from build123d import *

# Parameters (mm, degrees)
BOSS_EXTRUDE1_DEPTH           = 17
CUT_EXTRUDE1_DEPTH            = 17
SKETCH3_R                     = 1.25
CUT_EXTRUDE2_DEPTH            = 17
CUT_EXTRUDE3_START            = -10.402815
SKETCH4_W                     = 3.3
SKETCH4_H                     = 12.499682623
CUT_EXTRUDE3_DEPTH            = 10.402815
SKETCH5_R                     = 2.25
SKETCH5_R_2                   = 1.25
EXTRUDE_THIN1_DEPTH           = 1.65
EXTRUDE_THIN1_TAPER           = -30
EXTRUDE_THIN1_OTHER_WAY_DEPTH = 1.65
EXTRUDE_THIN1_OTHER_WAY_TAPER = -30
SKETCH6_R                     = 1.25
CUT_EXTRUDE4_DEPTH            = 58.713758796
CUT_EXTRUDE5_DEPTH            = 47
CUT_EXTRUDE6_DEPTH            = 51
SKETCH9_R                     = 4
CUT_EXTRUDE7_DEPTH            = 51
CHAMFER2_SIZE                 = 4
CHAMFER2_SIZE_2               = 0.5
FILLET3_R                     = 30
FILLET4_SIZE                  = 2
FILLET4_SIZE_2                = 10


with BuildPart() as part:
    # Sketch1 → Boss-Extrude1 (new body)
    with BuildSketch(Plane.XY):
        Polygon((0, 0), (-3.159113316, 10.05), (-6.746853749, 9.105426772), (-9.395430715, 19.165426772), (-16.396843313, 17.322108667), (-13.748266347, 7.262108667), (-16.987870242, 6.409192141), (-13.249821349, -13.430807859), (-10.069194805, -33.377281726), (4.664340434, -45.432247006), (8.210516928, -41.098122841), (1.353313338, -35.487565032), (13.657279278, -20.449702081), (20.514482868, -26.06025989), (24.060659362, -21.726135725), (15.88, -15.032727593), align=None)
    extrude(amount=BOSS_EXTRUDE1_DEPTH)

    # Sketch2 → Cut-Extrude1 (cut)
    with BuildSketch(Plane(origin=(-11.069057434, -2.914239618, 0), x_dir=(0, 0, 1), z_dir=(-0.9670459389139427, -0.2546019482055291, 0))):
        with BuildLine():
            Line((14.33099337, 13.694095472), (13.19, 10.523128091))
            Line((13.19, 10.523128091), (20.415721384, 10.523128091))
            Line((20.415721384, 10.523128091), (20.415721384, 21.928823046))
            Line((20.415721384, 21.928823046), (-2.093019815, 21.928823046))
            Line((-2.093019815, 21.928823046), (-2.093019815, 20.981086575))
            Line((-2.093019815, 20.981086575), (9.161350785, 20.925943092))
            ThreePointArc((9.161350785, 20.925943092), (13.295140538, 18.417290029), (14.33099337, 13.694095472))
        make_face()
    extrude(amount=-CUT_EXTRUDE1_DEPTH, mode=Mode.SUBTRACT)

    # Sketch3 → Cut-Extrude2 (cut)
    with BuildSketch(Plane(origin=(-11.069057434, -2.914239618, 0), x_dir=(0, 0, 1), z_dir=(-0.9670459389139427, -0.2546019482055291, 0))):
        with Locations(Location((8.8, 16.925943092, 0), (0, 0, 270))):
            Circle(SKETCH3_R)
    extrude(amount=-CUT_EXTRUDE2_DEPTH, mode=Mode.SUBTRACT)

    # Sketch4 → Cut-Extrude3 (cut)
    with BuildSketch(Plane(origin=(-5.327785879, 20.236348285, 0), x_dir=(0.9670459389139427, 0.2546019482055291, 0), z_dir=(-0.2546019482055291, 0.9670459389139427, 0)).offset(CUT_EXTRUDE3_START)):
        with Locations((-7.826258123, -8.749841312)):
            Rectangle(SKETCH4_W, SKETCH4_H)
    extrude(amount=CUT_EXTRUDE3_DEPTH, mode=Mode.SUBTRACT)

    # Sketch5 → Extrude-Thin1 (add)
    with BuildSketch(Plane(origin=(-7.568351135, -1.992580565, 0), x_dir=(0, 0, 1), z_dir=(-0.9670459389139427, -0.25460194820552917, 0))):
        with Locations((8.8, 16.925943092)):
            Circle(SKETCH5_R)
        with Locations((8.8, 16.925943092)):
            Circle(SKETCH5_R_2, mode=Mode.SUBTRACT)
    extrude(amount=EXTRUDE_THIN1_DEPTH, taper=EXTRUDE_THIN1_TAPER)

    # Sketch5 → Extrude-Thin1 other way (add)
    with BuildSketch(Plane(origin=(-7.568351135, -1.992580565, 0), x_dir=(0, 0, 1), z_dir=(-0.9670459389139427, -0.25460194820552917, 0))):
        with Locations((8.8, 16.925943092)):
            Circle(SKETCH5_R)
        with Locations((8.8, 16.925943092)):
            Circle(SKETCH5_R_2, mode=Mode.SUBTRACT)
    extrude(amount=-EXTRUDE_THIN1_OTHER_WAY_DEPTH, taper=EXTRUDE_THIN1_OTHER_WAY_TAPER)

    # Sketch6 → Cut-Extrude4 (cut, through all)
    with BuildSketch(Plane(origin=(-11.069057434, -2.914239618, 0), x_dir=(0, 0, 1), z_dir=(-0.9670459389139427, -0.2546019482055291, 0))):
        with Locations(Location((8.8, 16.925943092, 0), (0, 0, 270))):
            Circle(SKETCH6_R)
    extrude(amount=-CUT_EXTRUDE4_DEPTH, mode=Mode.SUBTRACT)

    # Sketch7 → Cut-Extrude5 (cut)
    with BuildSketch(Plane(origin=(-20.395990741, -24.927906579, 0), x_dir=(-0.773950743756153, 0.633245802385849, 0), z_dir=(-0.6332458023858489, -0.7739507437561529, 0))):
        with BuildLine():
            add(Edge.make_bspline(
                [(-28.329749458, 0), (-30.166192179, -1.367621789), (-30.599748983, -3.6)],
                knots=[0, 0, 0, 1, 1, 1], degree=2))
            Line((-28.329749458, 0), (-32.379749458, 0))
            Line((-32.379749458, 0), (-32.379749458, -17))
            Line((-32.379749458, -17), (-30.599749458, -17))
            Line((-30.599749458, -17), (-30.599749458, -13.1))
            ThreePointArc((-30.599749458, -13.1), (-31.973295872, -8.349999931), (-30.599748983, -3.6))
        make_face()
    extrude(amount=-CUT_EXTRUDE5_DEPTH, mode=Mode.SUBTRACT)

    # Sketch8 → Cut-Extrude6 (cut)
    with BuildSketch(Plane(origin=(-4.545848307, -5.555919463, 0), x_dir=(0.7739507437561534, -0.6332458023858486, 0), z_dir=(-0.6332458023858486, -0.7739507437561534, 0))):
        with BuildLine():
            Line((30.599749458, 13.1), (30.599749458, 17))
            Line((30.599749458, 17), (23.519749458, 17))
            ThreePointArc((23.519749458, 17), (27.561296191, 15.960500224), (30.599749458, 13.1))
        make_face()
    extrude(amount=-CUT_EXTRUDE6_DEPTH, mode=Mode.SUBTRACT)

    # Sketch9 → Cut-Extrude7 (cut)
    with BuildSketch(Plane(origin=(-20.395990741, -24.927906579, 0), x_dir=(-0.773950743756153, 0.633245802385849, 0), z_dir=(-0.6332458023858489, -0.7739507437561529, 0))):
        with Locations(Location((-26.599749458, -8.5, 0), (0, 0, 180))):
            Circle(SKETCH9_R)
    extrude(amount=-CUT_EXTRUDE7_DEPTH, mode=Mode.SUBTRACT)

    # Chamfer2
    # the kernel refuses this chamfer: 4, 0.5 mm, written as the material it takes off along each edge
    with BuildSketch(Plane(origin=(23.430476857, -22.180351132, 17), x_dir=(0.003280548241470475, 0.003465446024389789, -0.9999886142787264), z_dir=(-0.7262148132107521, 0.6874678502106645, 0))) as chamfer2_piece_1_section:
        Polygon((CHAMFER2_SIZE * 0.999988614279, CHAMFER2_SIZE * 0.00477192968437), (-CHAMFER2_SIZE_2 * 0.00477192968437, CHAMFER2_SIZE_2 * 0.999988614279), (0, 0), align=None)
    chamfer2_piece_1 = extrude(amount=42.660867212, mode=Mode.PRIVATE)
    chamfer2_piece_1 = split(chamfer2_piece_1, bisect_by=Plane(origin=(2.714923218, -8.636910301, 15.455863369), z_dir=(0.9539790028805075, 0.2998734100635013, 0)), keep=Keep.TOP, mode=Mode.PRIVATE)
    chamfer2_piece_1 = split(chamfer2_piece_1, bisect_by=Plane(origin=(6.949444097, -7.725754787, 15.455863369), z_dir=(0.6332458023858455, 0.7739507437561558, 0)), keep=Keep.TOP, mode=Mode.PRIVATE)
    add(chamfer2_piece_1, mode=Mode.SUBTRACT)
    with BuildSketch(Plane(origin=(3.117792699, -9.918547862, 17), x_dir=(0.0045523207221114005, 0.0014309748270353465, -0.9999886142787264), z_dir=(-0.2998734100635013, 0.9539790028805075, 0))) as chamfer2_piece_2_section:
        Polygon((CHAMFER2_SIZE * 0.999988614279, CHAMFER2_SIZE * 0.00477192968437), (-CHAMFER2_SIZE_2 * 0.00477192968437, CHAMFER2_SIZE_2 * 0.999988614279), (0, 0), align=None)
    chamfer2_piece_2 = extrude(amount=31.328882119, mode=Mode.PRIVATE)
    chamfer2_piece_2 = split(chamfer2_piece_2, bisect_by=Plane(origin=(-6.749370263, 6.389259735, 15.513791759), z_dir=(0.6874678502106645, 0.7262148132107521, 0)), keep=Keep.TOP, mode=Mode.PRIVATE)
    add(chamfer2_piece_2, mode=Mode.SUBTRACT)
    with BuildSketch(Plane(origin=(3.117792699, -9.918547862, 17), x_dir=(0.0045523207221114005, 0.0014309748270353465, -0.9999886142787264), z_dir=(-0.2998734100635013, 0.9539790028805075, 0))) as chamfer2_piece_3a_section:
        Polygon((CHAMFER2_SIZE * 0.999988614279, CHAMFER2_SIZE * 0.00477192968437), (-CHAMFER2_SIZE_2 * 0.00477192968437, CHAMFER2_SIZE_2 * 0.999988614279), (0, 0), align=None)
    chamfer2_piece_3a = extrude(amount=31.328882119, mode=Mode.PRIVATE)
    chamfer2_piece_3a = split(chamfer2_piece_3a, bisect_by=Plane(origin=(3.183687603, -3.013822952, 15.535130807), z_dir=(-0.6874678502106645, -0.7262148132107521, 0)), keep=Keep.TOP, mode=Mode.PRIVATE)
    with BuildSketch(Plane(origin=(23.430476857, -22.180351132, 17), x_dir=(0.003280548241470475, 0.003465446024389789, -0.9999886142787264), z_dir=(-0.7262148132107521, 0.6874678502106645, 0))) as chamfer2_piece_3b_section:
        Polygon((CHAMFER2_SIZE * 0.999988614279, CHAMFER2_SIZE * 0.00477192968437), (-CHAMFER2_SIZE_2 * 0.00477192968437, CHAMFER2_SIZE_2 * 0.999988614279), (0, 0), align=None)
    chamfer2_piece_3b = extrude(amount=42.660867212, mode=Mode.PRIVATE)
    chamfer2_piece_3b = split(chamfer2_piece_3b, bisect_by=Plane(origin=(-1.314629282, 4.18219385, 15.535130807), z_dir=(-0.9539790028805075, -0.2998734100635013, 0)), keep=Keep.TOP, mode=Mode.PRIVATE)
    chamfer2_piece_3 = chamfer2_piece_3a & chamfer2_piece_3b
    add(chamfer2_piece_3, mode=Mode.SUBTRACT)

    # Fillet3
    # the kernel refuses this fillet: 30 mm, written as the material it adds along each edge
    with BuildSketch(Plane(origin=(19.498535053, -17.993409719, 10.299717624), x_dir=(0.3870758506648627, -0.3167051128458923, 0.865950435838763), z_dir=(-0.6702029838732583, 0.5483594785692364, 0.500129825815914))) as fillet3_piece_1_section:
        with BuildLine():
            CenterArc((FILLET3_R * 0.071988838012, FILLET3_R), FILLET3_R, 261.764893066, 8.235106934)
            Line((-FILLET3_R * 0.071246536041, FILLET3_R * 0.0103113481403), (0, 0))
            Line((0, 0), (FILLET3_R * 0.071988838012, 0))
        make_face()
    fillet3_piece_1 = extrude(amount=18.796249028, mode=Mode.PRIVATE)
    fillet3_piece_1 = split(fillet3_piece_1, bisect_by=Plane(origin=(13.825719707, -13.08805278, 14.411900392), z_dir=(-0.6874678502106645, -0.7262148132107521, 0)), keep=Keep.TOP, mode=Mode.PRIVATE)
    fillet3_piece_1 = split(fillet3_piece_1, bisect_by=Plane(origin=(13.532386136, -13.397919176, 17), z_dir=(0, 0, -1)), keep=Keep.TOP, mode=Mode.PRIVATE)
    fillet3_piece_1 = fillet3_piece_1 - Plane(origin=(19.447051663, -18.23729319, 8.5), x_dir=(0.773950743756153, -0.633245802385849, 0), z_dir=(-0.633245802385849, -0.773950743756153, 0)) * Cylinder(4, 47, mode=Mode.PRIVATE)
    add(fillet3_piece_1)

    # Fillet4
    # an asymmetric fillet: 10, 2 mm, written as the material it takes off along each edge
    with BuildSketch(Plane(origin=(14.780717757, 25.530475477, 0), x_dir=(0.2546019482055286, -0.9670459389139429, 0), z_dir=(-0.9670459389139429, -0.2546019482055286, 0))) as fillet4_piece_1:
        with BuildLine():
            Bezier((FILLET4_SIZE, 0), (0, 0), (0, FILLET4_SIZE_2), weights=[1, 0.707106781, 1])
            Line((0, FILLET4_SIZE_2), (0, 0))
            Line((0, 0), (FILLET4_SIZE, 0))
        make_face()
    extrude(amount=57.24, mode=Mode.SUBTRACT)


solid = part.part
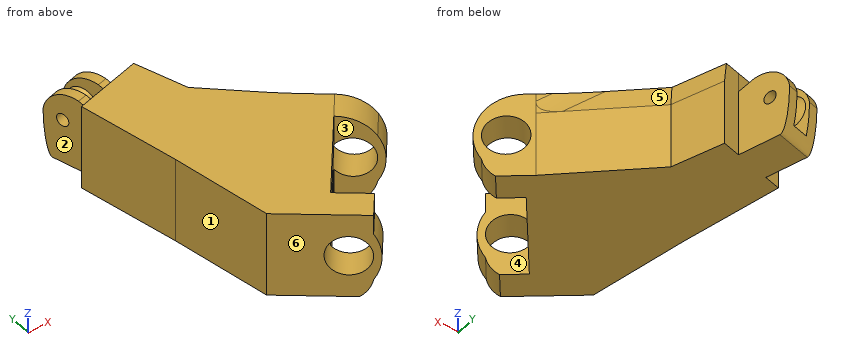
The listing builds one solid part. Answer for the finished solid, in the listing's coordinates (mm). Face numbers are marked on the shaded views. A direction names the side the tool comes from. Coordinates: 2 decimals unless noted, no trailing zeros. Order: outer loops, then holes, each group sorted by start corner. A loop starts at its lowest first (then second) coordinate and runs counter-clockwise, first axis right, second up. Notation, with made-up numbers: (-16, -39.75) -> (-6, -39.75) arc R10 ccw to (-6, -33.75) -> close; hole circle Ø5 at (67, 41). An arc over 180 degrees is marked (long way). Answer in a Markdown table with one row per item. Add a question column.
Item 1: Each of these flat-tipped pins is pushed along its axis until it touches: P1, Ø6, axis at x = -12, z = 9, coming from the -Y side; P2, Ø10, axis at x = 18, z = 5.5, coming from the +Y side; P3, Ø1.7, axis at x = -11.5, y = 12.5, coming from the +Z side; P4, Ø2, axis at x = -8, y = -38.5, coming from the +Z side. Where does it stop, or does it pass through?
Item 2: Find section A-A (y = 2). Write down the section's boundary in (x, z), then the cut area to 3 significant figures.
Item 3: Which of the six approach directions +Z, -Z, +X, -X, +Y, -Y give full straight-line access (tool end or side, diameter ignored) to the marked faces 1, 2 and 3?
Item 4: Determine the mould class of the marked faces 4, 5 and 6 for opening direction Y: +Y half, -Y half, draft (parallel to the pull), parting line (faces both ways), or undercut.
Item 5: Find section B-B (y = -5). Write down the section's boundary in (x, z).
Item 6: Find the intervals of material crossed by L1, parallel to Y at x = 6, z = 7.25; L2, parallel to X at y = 10.5, z = 9.5; L3, parallel to X at y = -24.5, z = 3.5, in increasing order. Write a range as from..to.
Result set:
| question | item | result |
|---|---|---|
| 1 | P1 | stops at y = -34.25 |
| 1 | P2 | stops at y = -12.31 |
| 1 | P3 | stops at z = 11.12 |
| 1 | P4 | passes through |
| 2 | outline | (-16.16, 0) -> (-0.63, 0) -> (-0.63, 13) -> (-1.15, 17) -> (-16.16, 17) -> close |
| 2 | area | 263 mm² |
| 3 | face 1 | +Z, -Z, -X, -Y |
| 3 | face 2 | +Z, -Z, -X |
| 3 | face 3 | +Z, -Z, -Y |
| 4 | face 4 | undercut |
| 4 | face 5 | +Y half |
| 4 | face 6 | -Y half |
| 5 | outline | (-14.84, 0) -> (5.28, 0) -> (5.28, 13) -> (4.55, 17) -> (-14.84, 17) -> close |
| 6 | L1 | y = -43.05..-40.67, -28.67..-5.68 |
| 6 | L2 | x = -14.6..-12.56, -9.15..-7.11 |
| 6 | L3 | x = -11.48..10.34, 18.61..19.47 |
